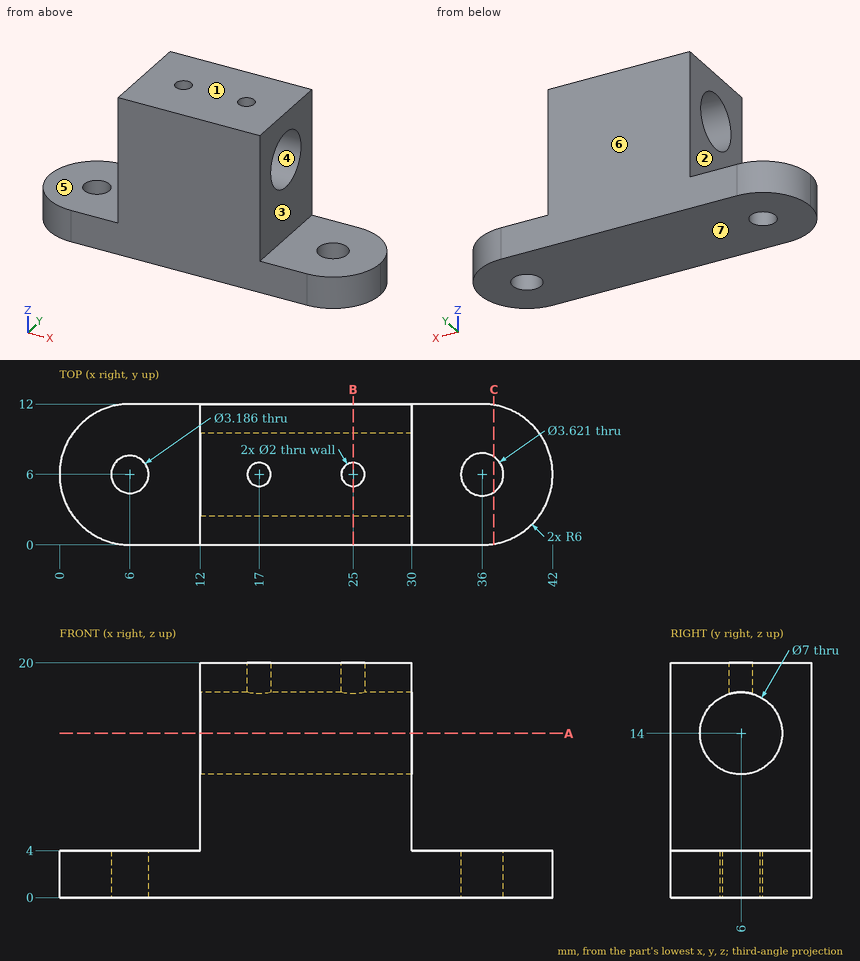
For this review, use the dimensioned drawing (mm, ordinates from the lowest corner) and the shaded views. A direction names the side the tool comes from. Coordinates: 2 decimals unless noted, no trailing zeros. Order: outer loops, then holes, each group sorted by start corner. A loop starts at its lowest first (then second) coordinate and runs counter-clockwise, first axis right, second up. Notation, with made-up numbers: (-8, 18.5) -> (51, 18.5) arc R19 ccw to (51, 28.5) -> close; hole circle Ø11 at (35, -22). An arc over 180 degrees is marked (long way). One line per item, written item: value. Start each with the question number.
Q1. Take a section at C-C, the plane x = 37. State the section outline as (y, z) points.
Q2. Tool access review of the marked faces 1, 2 and 3: name each direction out of +Z, -Z, +X, -X, +Y, -Y from which nothing blocks a thin tool from reaching the whole face with its end or side.
Q3. Mouldability with a two-part tool opening along Z and no side actions: class the marked faces 4, 5, 6 and 7 as pulls with the +Z half, pulls with the -Z half, needs draft (parallel to the pull), parting line crosses it, or undercut.
Q4. For probe 1 along Z at (x, y) = (23, 6.25); probe 2 along X at (y, z) = (6.75, 18.75); probe 3 along Y at (x, z) = (17, 18.4), list the stretches that pass through material, from the lowest coordinate up.
Q5. Insertion check: pin 1 Ø4 at (x, y) = (36, 6) entering from -Z; pin 2 Ø6 at (y, z) = (7.5, 17) entering from -X; pin 3 Ø3.5 at (x, y) = (6, 6) entering from +Z; pin 4 Ø1.5 at (y, z) = (5.5, 17) entering from +X. Each pin has a flat end and moves straight along its axis. Give the tip position at first contact, or say it passes through.
Q6. Take a section at B-B, the plane x = 25. State the section outline as (y, z) points.
Q7. Take a section at A-A, the plane z = 14. State the section outline as (x, y) points, then the cut area to 3 significant figures.
Values follow:
1. outline: (0.08, 0) -> (4.49, 0) -> (4.49, 4) -> (0.08, 4) -> close; (7.51, 0) -> (11.92, 0) -> (11.92, 4) -> (7.51, 4) -> close
2. face 1: +Z, +X, -X, +Y, -Y
2. face 2: +Z, -X, +Y, -Y
2. face 3: +Z, +X, +Y, -Y
3. face 4: undercut
3. face 5: pulls with the +Z half
3. face 6: needs draft
3. face 7: pulls with the -Z half
4. probe 1: z = 0 to 10.51, 17.49 to 20
4. probe 2: x = 12 to 16.34, 17.66 to 24.34, 25.66 to 30
4. probe 3: y = 0 to 5, 7 to 12
5. pin 1: stops at z = 0
5. pin 2: stops at x = 12
5. pin 3: stops at z = 4
5. pin 4: stops at x = 30
6. outline: (0, 0) -> (12, 0) -> (12, 20) -> (7, 20) -> (7, 17.35) arc R3.5 cw (long way) to (5, 17.35) -> (5, 20) -> (0, 20) -> close
7. outline: (12, 0) -> (30, 0) -> (30, 2.5) -> (12, 2.5) -> close; (12, 9.5) -> (30, 9.5) -> (30, 12) -> (12, 12) -> close
7. area: 90.0 mm2
